from build123d import *

# Parameters (mm, degrees)
SKETCH_1_W          = 30
SKETCH_1_H          = 15
EXTRUDE_1_DEPTH     = 5
SKETCH_2_W          = 10
SKETCH_2_H          = 5.85548899
EXTRUDE_3_DEPTH     = 10
SKETCH_4_R          = 1.5
CUT_EXTRUDE_1_DEPTH = 6
SKETCH_5_R          = 1.5
CUT_EXTRUDE_2_DEPTH = 5


with BuildPart() as part:
    # Эскиз1 → Бобышка-Вытянуть1 (new body)
    with BuildSketch(Plane(origin=(0, 0, 0), x_dir=(1, 0, 0), z_dir=(0, 1, 0))):
        with Locations((-25.518864851, -20.257046334)):
            Rectangle(SKETCH_1_W, SKETCH_1_H)
    extrude(amount=EXTRUDE_1_DEPTH)

    # Эскиз2 → Бобышка-Вытянуть3 (add)
    with BuildSketch(Plane(origin=(0, 5, 0), x_dir=(1, 0, 0), z_dir=(0, 1, 0))):
        with Locations((-20.518864851, -15.684790829)):
            Rectangle(SKETCH_2_W, SKETCH_2_H)
        with Locations((-30.518864851, -15.684790829)):
            Rectangle(SKETCH_2_W, SKETCH_2_H)
    extrude(amount=EXTRUDE_3_DEPTH)

    # Эскиз4 → Вырез-Вытянуть1 (cut)
    with BuildSketch(Plane.XY.offset(18.612535324)):
        with Locations((-20.518864851, 10)):
            Circle(SKETCH_4_R)
        with Locations((-30.518864851, 10)):
            Circle(SKETCH_4_R)
    extrude(amount=-CUT_EXTRUDE_1_DEPTH, mode=Mode.SUBTRACT)

    # Эскиз5 → Вырез-Вытянуть2 (cut)
    with BuildSketch(Plane(origin=(0, 5, 0), x_dir=(1, 0, 0), z_dir=(0, 1, 0))):
        with Locations(Location((-34.518864851, -23.184790829, 0), (0, 0, 270))):
            Circle(SKETCH_5_R)
        with Locations(Location((-16.518864851, -23.184790829, 0), (0, 0, 270))):
            Circle(SKETCH_5_R)
    extrude(amount=-CUT_EXTRUDE_2_DEPTH, mode=Mode.SUBTRACT)


solid = part.part
Read the model definition and answer for the solid it produces. Units are mm, in the model's axes. A direction names the side the tool comes from. Round coordinates to 2 decimals unless told otherwise and drop trailing zeros. Write each loop counter-clockwise with the first axis right and the second up, starting at its lowest first coordinate (ties: lowest second). Pieces come first, ordered by that corner, then holes.
Q1. The mould has two halves that part along Z. Classify faces 1 (the face through (-34.068, 2.535, 24.616)), 2 (the face through (-26, 5, 22)), 3 (the face through (-26, 10, 18.613)): released by +Z, released by -Z, zero draft, split by the parting line, or undercut.
Values:
face 1: undercut
face 2: zero draft
face 3: released by +Z
Q2. Find section A-A on y = 10. Determine the outline of the cut face in (x, z).
Values:
outline: (-35.52, 12.76) - (-32.02, 12.76) - (-32.02, 18.61) - (-35.52, 18.61) - close; (-29.02, 12.76) - (-22.02, 12.76) - (-22.02, 18.61) - (-29.02, 18.61) - close; (-19.02, 12.76) - (-15.52, 12.76) - (-15.52, 18.61) - (-19.02, 18.61) - close
Q3. Find section B-B on z = 24. Determine the outline of the cut face in (x, y), and give its area (3 significant figures).
Values:
outline: (-40.52, 0) - (-35.78, 0) - (-35.78, 5) - (-40.52, 5) - close; (-33.26, 0) - (-17.78, 0) - (-17.78, 5) - (-33.26, 5) - close; (-15.26, 0) - (-10.52, 0) - (-10.52, 5) - (-15.26, 5) - close
area: 125 mm2
Q4. Flat-ended cylindrical pins translate along their axes: P1, Ø3, axis at y = 12, z = 16, coming from the -X side; P2, Ø4.5, axis at x = -31.5, z = 20, coming from the +Y side; P3, Ø1.5, axis at x = -35, y = 7, coming from the +Z side; P4, Ø2.5, axis at x = -34.52, z = 23.18, coming from the +Y side. Find the tip coordinate at first contact, or state that the pin passes through.
Values:
P1: stops at x = -35.52
P2: stops at y = 15
P3: stops at z = 18.61
P4: passes through
Q5. Find section D-D on z = 14. Determine the outline of the cut face in (x, y).
Values:
outline: (-40.52, 0) - (-10.52, 0) - (-10.52, 5) - (-15.52, 5) - (-15.52, 15) - (-35.52, 15) - (-35.52, 5) - (-40.52, 5) - close; hole circle Ø3 at (-30.52, 10); hole circle Ø3 at (-20.52, 10)
Q6. A tool of negligible diameter and unlimited length cuts with its end or side. For faces 4 (the face through (-15.519, 10, 16)), 5 (the face through (-26, 2, 27.757)), 6 (the face through (-35.519, 10, 16)), from which of +Z, -Z, +X, -X, +Y, -Y can it reach the whole face along a straight path? Write none if from no direction.
Values:
face 4: +Z, -Z, +X, +Y
face 5: +Z, +X, -X, +Y, -Y
face 6: +Z, -Z, -X, +Y
Q7. Straight lines are drawn through the part: line 1 (X direction, y = 4.75, z = 23.25); line 2 (X direction, y = 1.25, z = 22); line 3 (Y direction, x = -19, z = 19). For each, find the intervals that lie inside material, in ascending order.
Values:
line 1: x = -40.52 to -36.02, -33.02 to -18.02, -15.02 to -10.52
line 2: x = -40.52 to -35.44, -33.6 to -17.44, -15.6 to -10.52
line 3: y = 0 to 5
Q8. Find section C-C on x = -20. Determine the outline of the cut face in (y, z), and give its area (3 significant figures).
Values:
outline: (0, 12.76) - (8.59, 12.76) - (8.59, 18.61) - (5, 18.61) - (5, 27.76) - (0, 27.76) - close; (11.41, 12.76) - (15, 12.76) - (15, 18.61) - (11.41, 18.61) - close
area: 117 mm2
